```python
from build123d import *

# Parameters (mm, degrees)
F0_W     = 30
F0_H     = 34.5
F1_DEPTH = 12.7
F2_R     = 2.47581
F2_R_2   = 2.592186
F2_R_3   = 2.442266
F2_R_4   = 2.394142
F3_DEPTH = 12.701
F4_R     = 1.5
F5_R     = 4.1
F6_DEPTH = 34.501


with BuildPart() as f1:
    # F0 (on Front) → F1 (new body)
    with BuildSketch(Plane.XZ):
        Rectangle(F0_W, F0_H)
    extrude(amount=F1_DEPTH)

    # F2 (on face) → F3 (cut, through all)
    with BuildSketch(Plane.XZ.offset(12.7)):
        with Locations((-9, 12)):
            Circle(F2_R)
        with Locations((-9, -12)):
            Circle(F2_R_2)
        with Locations((9, 12)):
            Circle(F2_R_3)
        with Locations((9, -12)):
            Circle(F2_R_4)
    extrude(amount=-F3_DEPTH, mode=Mode.SUBTRACT)

    # F4
    f4_edges = [f1.edges().sort_by_distance(p)[0] for p in [
        (-15, 0, 0),
        (0, 0, 17.25),
        (15, 0, 0),
        (0, 0, -17.25),
        (15, -12.7, 0),
        (0, -12.7, 17.25),
        (-15, -12.7, 0),
        (0, -12.7, -17.25),
    ]]
    fillet(f4_edges, radius=F4_R)

    # F5 (on face) → F6 (cut, through all)
    with BuildSketch(Plane(origin=(0, 0, -17.25), x_dir=(1, 0, 0), z_dir=(0, 0, -1))):
        with Locations((0, 6.991122)):
            Circle(F5_R)
    extrude(amount=-F6_DEPTH, mode=Mode.SUBTRACT)


solid = f1.part
```
Work out the finished part from the listing and answer in its coordinate system (mm). Coordinates: 2 decimals unless noted, no trailing zeros. Write each loop counter-clockwise with the first axis right and the second up, starting at its lowest first coordinate (ties: lowest second). Pieces come first, ordered by that corner, then holes.
Q1. Determine the mould class of faces 1 (the face through (8.481, -6.439, -14.337)), 2 (the face through (-6.605, -6.439, -12.993)), 3 (the face through (-14.57, -12.25, 0.24)), 4 (the face through (0.21, -0.45, 16.82)) for opening direction Z: released by +Z, released by -Z, zero draft, split by the parting line, or undercut.
Q2. A cutting plane is placed at A-A, the plane x = -9. Give the vertices of the cut face in (y, z), then the cut area to 3 significant figures.
Q3. A cutting plane is placed at C-C, the plane x = 0. Give the vertices of the cut face in (y, z).
Q4. A cutting plane is placed at B-B, the plane y = -5. Give the vertices of the cut face in (x, z), then the cut area to 3 significant figures.
Q5. Find the intervals of material crossed by line 1 (Z direction, x = 9, y = -3.5); line 2 (Z direction, x = -9, y = -10); line 3 (X direction, y = -2.75, z = 14), in increasing order.
Q6. This flat-tipped pin is pushed along its axis until it touches: pin 1 Ø3 at (x, z) = (-9, 12) entering from +Y. Where does it stop, or does it pass through?
Q7. A cutting plane is placed at D-D, the plane z = 9. Give the vertices of the cut face in (x, y), then the cut area to 3 significant figures.
Findings below:
1. face 1: undercut
1. face 2: undercut
1. face 3: zero draft
1. face 4: released by +Z
2. outline: (-12.7, -15.75) arc R1.5 ccw to (-11.2, -17.25) - (-1.5, -17.25) arc R1.5 ccw to (0, -15.75) - (0, -14.59) - (-12.7, -14.59) - close; (-12.7, -9.41) - (0, -9.41) - (0, 9.52) - (-12.7, 9.52) - close; (-12.7, 14.48) - (0, 14.48) - (0, 15.75) arc R1.5 ccw to (-1.5, 17.25) - (-11.2, 17.25) arc R1.5 ccw to (-12.7, 15.75) - close
2. area: 307 mm2
3. outline: (-12.7, -15.75) arc R1.5 ccw to (-11.2, -17.25) - (-11.09, -17.25) - (-11.09, 17.25) - (-11.2, 17.25) arc R1.5 ccw to (-12.7, 15.75) - close; (-2.89, -17.25) - (-1.5, -17.25) arc R1.5 ccw to (0, -15.75) - (0, 15.75) arc R1.5 ccw to (-1.5, 17.25) - (-2.89, 17.25) - close
4. outline: (-15, -17.25) - (-3.58, -17.25) - (-3.58, 17.25) - (-15, 17.25) - close; (3.58, -17.25) - (15, -17.25) - (15, 17.25) - (3.58, 17.25) - close; hole circle Ø5.18 at (-9, -12); hole circle Ø4.95 at (-9, 12); hole circle Ø4.88 at (9, 12); hole circle Ø4.79 at (9, -12)
4. area: 711 mm2
5. line 1: z = -17.25 to -14.39, -9.61 to 9.56, 14.44 to 17.25
5. line 2: z = -17.25 to -14.59, -9.41 to 9.52, 14.48 to 17.25
5. line 3: x = -15 to -10.46, -7.54 to 7.6, 10.4 to 15
6. pin 1: passes through
7. outline: (-15, -11.2) arc R1.5 ccw to (-13.5, -12.7) - (13.5, -12.7) arc R1.5 ccw to (15, -11.2) - (15, -1.5) arc R1.5 ccw to (13.5, 0) - (-13.5, 0) arc R1.5 ccw to (-15, -1.5) - close; hole circle Ø8.2 at (0, -6.99)
7. area: 326 mm2
